```python
from build123d import *

# Parameters (mm, degrees)
SALIENTE_EXTRUIR1_DEPTH = 1
CROQUIS2_W              = 0.64
CROQUIS2_H              = 0.64
SALIENTE_EXTRUIR2_DEPTH = 5.6
CHAFL_N1_SIZE           = 0.1
CHAFL_N1_SIZE2          = 0.567128182
CHAFL_N1_PART_2_SIZE    = 0.1
CHAFL_N1_PART_2_SIZE2   = 0.567128182


with BuildPart() as part:
    # Croquis1 → Saliente-Extruir1 (new body, symmetric)
    with BuildSketch(Plane(origin=(0, 0, 0), x_dir=(1, 0, 0), z_dir=(0, 1, 0))):
        Polygon((-1.27, 0.92), (-0.92, 1.27), (0.92, 1.27), (1.27, 0.92), (1.27, -0.92), (0.92, -1.27), (-0.92, -1.27), (-1.27, -0.92), align=None)
    extrude(amount=SALIENTE_EXTRUIR1_DEPTH, both=True)

    # Croquis2 → Saliente-Extruir2 (add, symmetric)
    with BuildSketch(Plane(origin=(0, 0, 0), x_dir=(1, 0, 0), z_dir=(0, 1, 0))):
        Rectangle(CROQUIS2_W, CROQUIS2_H)
    extrude(amount=SALIENTE_EXTRUIR2_DEPTH, both=True)

    # Chaflán1
    chafl_n1_edges = [part.edges().sort_by_distance(p)[0] for p in [
        (0.32, -5.6, 0),
        (0, -5.6, -0.32),
        (-0.32, -5.6, 0),
        (0, -5.6, 0.32),
    ]]
    chafl_n1_side = [part.faces().sort_by_distance(p)[0] for p in [
        (0, -5.6, 0),
    ]]
    chamfer(chafl_n1_edges, length=CHAFL_N1_SIZE, length2=CHAFL_N1_SIZE2, reference=chafl_n1_side[0])

    # Chaflán1 part 2
    chafl_n1_part_2_edges = [part.edges().sort_by_distance(p)[0] for p in [
        (0.32, 5.6, 0),
        (0, 5.6, -0.32),
        (-0.32, 5.6, 0),
        (0, 5.6, 0.32),
    ]]
    chafl_n1_part_2_side = [part.faces().sort_by_distance(p)[0] for p in [
        (0, 5.6, 0),
    ]]
    chamfer(chafl_n1_part_2_edges, length=CHAFL_N1_PART_2_SIZE, length2=CHAFL_N1_PART_2_SIZE2, reference=chafl_n1_part_2_side[0])


solid = part.part
```
Read the model definition and answer for the solid it produces. Units are mm, in the model's axes. A direction names the side the tool comes from. Coordinates: 2 decimals unless noted, no trailing zeros. Write each loop counter-clockwise with the first axis right and the second up, starting at its lowest first coordinate (ties: lowest second). Pieces come first, ordered by that corner, then holes. Notation, with made-up numbers: (72, 76.25) - (123, 76.25) arc R20 cw to (123, 102.25) - close; hole circle Ø4 at (-4.5, 63.25). An arc over 180 degrees is marked (long way). Answer as a JSON object with one key per item and string values. Group by question number.
1. Each of these flat-tipped pins is pushed along its axis until it touches: P1, Ø0.7, axis at x = 0, y = -2.5, coming from the -Z side; P2, Ø0.7, axis at x = 0, y = -4, coming from the +Z side; P3, Ø0.7, axis at y = 2, z = 0, coming from the -X side. Where does it stop, or does it pass through?
2. Which of the six approach directions +Z, -Z, +X, -X, +Y, -Y give full straight-line access (tool end or side, diameter ignored) to faces 1 (the flat face through (-1.27, 0, 0)), 2 (the flat face through (-1, -1, 0)), 3 (the flat face through (-1, 1, 0))?
3. Consider L1, parallel to X at y = -3, z = 0; L2, parallel to Y at x = -0.7, z = 0.05. Determine where each line is inside the solid, lowest interval first. Write a range as [from, to].
4. A cutting plane is placed at D-D (x = 1.1). Determine the outline of the cut face in (y, z), plus the area to 3 significant figures.
5. A cutting plane is placed at B-B (z = 0.1). Determine the outline of the cut face in (x, y), plus the area to 3 significant figures.
6. A cutting plane is placed at A-A (x = 0). Determine the outline of the cut face in (y, z), plus the area to 3 significant figures.
7. A cutting plane is placed at C-C (y = 0.25). Determine the outline of the cut face in (x, z), plus the area to 3 significant figures.
Worked out:
{
 "1": {"P1": "stops at z = -0.32", "P2": "stops at z = 0.32", "P3": "stops at x = -0.32"},
 "2": {"face 1": "+Z, -Z, -X, +Y, -Y", "face 2": "-Y", "face 3": "+Y"},
 "3": {"L1": "x = [-0.32, 0.32]", "L2": "y = [-1, 1]"},
 "4": {"outline": "(-1, -1.09) - (1, -1.09) - (1, 1.09) - (-1, 1.09) - close", "area": "4.36 mm²"},
 "5": {"outline": "(-1.27, -1) - (-0.32, -1) - (-0.32, -5.03) - (-0.22, -5.6) - (0.22, -5.6) - (0.32, -5.03) - (0.32, -1) - (1.27, -1) - (1.27, 1) - (0.32, 1) - (0.32, 5.03) - (0.22, 5.6) - (-0.22, 5.6) - (-0.32, 5.03) - (-0.32, 1) - (-1.27, 1) - close", "area": "10.9 mm²"},
 "6": {"outline": "(-5.6, -0.22) - (-5.03, -0.32) - (-1, -0.32) - (-1, -1.27) - (1, -1.27) - (1, -0.32) - (5.03, -0.32) - (5.6, -0.22) - (5.6, 0.22) - (5.03, 0.32) - (1, 0.32) - (1, 1.27) - (-1, 1.27) - (-1, 0.32) - (-5.03, 0.32) - (-5.6, 0.22) - close", "area": "10.9 mm²"},
 "7": {"outline": "(-1.27, -0.92) - (-0.92, -1.27) - (0.92, -1.27) - (1.27, -0.92) - (1.27, 0.92) - (0.92, 1.27) - (-0.92, 1.27) - (-1.27, 0.92) - close", "area": "6.21 mm²"}
}
